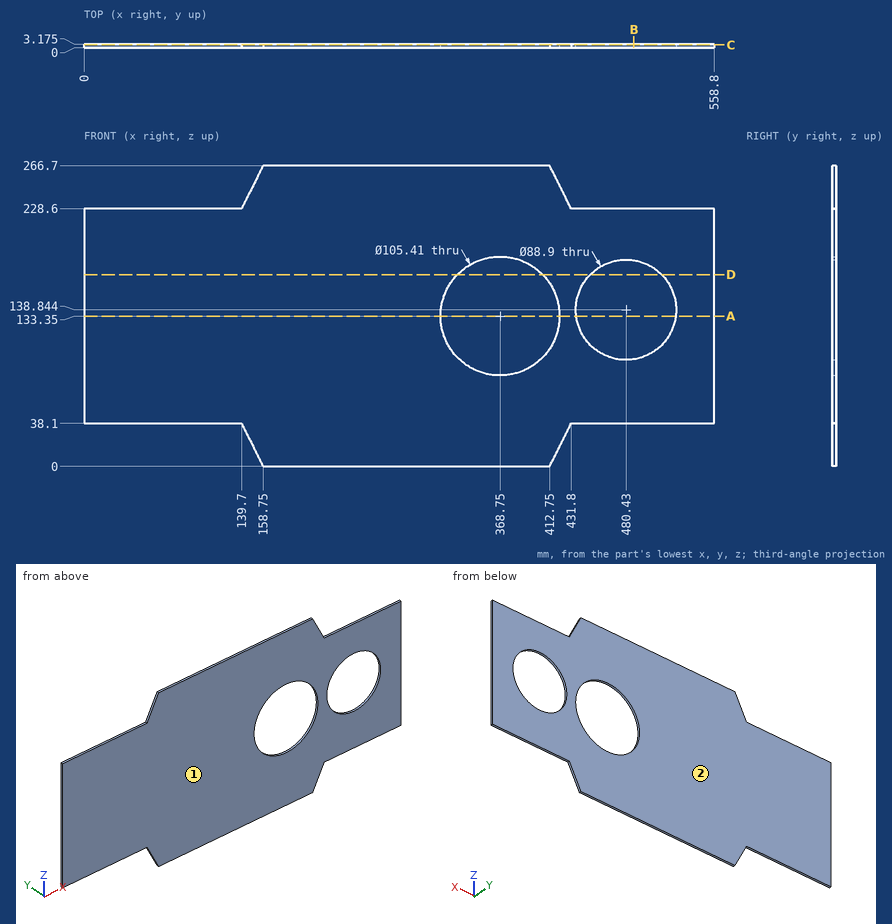
Could you check a few things on this drawing? It's one solid part, dimensions in mm from its lowest x, y, z. Coordinates: 2 decimals unless noted, no trailing zeros. Loops run counter-clockwise (first coordinate to the right, second up) from the corner with the lowest first, then second, coordinate; pieces in that order, holes last. Notation, with made-up numbers: (26.25, 27) - (64.25, 27) arc R22 cw to (64.25, 51) - close; hole circle Ø10 at (-25, 75). An arc over 180 degrees is marked (long way). Answer as a JSON object with one key per item and string values. Group by question number.
Item 1: If we section it at C-C (y = 2.3): State how many separate pieces and enclosed holes the cut face has, plus the area to 3 significant figures.
Item 2: If we section it at B-B (x = 487.5): List the corners of the cut face in (y, z) for me (1 decimal).
Item 3: If we mould it in two halves opening along Y, with no side actions, what happens to the marked faces 1 and 2? For each: released by +Y, released by -Y, zero draft, split by the parting line, or undercut.
Item 4: If we section it at D-D (z = 170): List the corners of the cut face in (x, y) for me (1 decimal).
Item 5: If I drill on L1, parallel to X at y = 1.8, z = 133.35 (1 decimal); L2, parallel to X at y = 1.3, z = 158 (1 decimal); L3, parallel to X at y = 2.7, z = 38, over which ranges is the centre line in solid material (lowest first)? Write a range as from..to.
Item 6: For pin 1 (1 mm diameter, centred on y = 0.5, z = 125, fed in from -X), with a flat end and sliding along its axis, tell me the tip position at first contact or that it passes through.
Item 7: If we section it at A-A (z = 133.35): List the corners of the cut face in (x, y) for me (1 decimal).
Returned:
{
 "1": {"separate pieces": "1", "enclosed holes": "2", "area": "112,000 mm²"},
 "2": {"outline": "(0, 38.1) - (3.2, 38.1) - (3.2, 95) - (0, 95) - close; (0, 182.7) - (3.2, 182.7) - (3.2, 228.6) - (0, 228.6) - close"},
 "3": {"face 1": "released by -Y", "face 2": "released by +Y"},
 "4": {"outline": "(0, 0) - (330.9, 0) - (330.9, 3.2) - (0, 3.2) - close; (406.6, 0) - (448.7, 0) - (448.7, 3.2) - (406.6, 3.2) - close; (512.1, 0) - (558.8, 0) - (558.8, 3.2) - (512.1, 3.2) - close"},
 "5": {"L1": "x = 0..316, 421.5..436.3, 524.5..558.8", "L2": "x = 0..322.2, 415.3..440.3, 520.5..558.8", "L3": "x = 139.75..431.75"},
 "6": {"pin 1": "stops at x = 0"},
 "7": {"outline": "(0, 0) - (316, 0) - (316, 3.2) - (0, 3.2) - close; (421.5, 0) - (436.3, 0) - (436.3, 3.2) - (421.5, 3.2) - close; (524.5, 0) - (558.8, 0) - (558.8, 3.2) - (524.5, 3.2) - close"}
}
